Autodesk Inventor part; units mm, degrees
ref_plane "Work Plane1" through (254, 0, 0) normal (1, 0, 0) x (0, 0, -1)
ref_plane "Work Plane2" through (254, 0, 0) normal (1, 0, 0) x (0, 0, -1)
ref_plane "Work Plane3" through (254, 0, 0) normal (1, 0, 0) x (0, 0, -1)
ref_plane "Work Plane1" through (254, 0, 0) normal (1, 0, 0) x (0, 0, -1)
ref_plane "Work Plane2" through (254, 0, 0) normal (1, 0, 0) x (0, 0, -1)
sketch "Sketch3" plane through (254, 0, 0) normal (1, 0, 0) x (0, 0, -1)
  arc A0 (-0.5014, 9.9874) -> (0.4986, 9.9876) centre (0, 0) ccw
  line L0 (0.4986, 9.9876) -> (-0.5014, 9.9874)
  line L1 (-0.5014, 9.9874) -> (-0.7511, 8.9686)
  line L2 (0.4986, 9.9876) -> (0.7489, 8.9688)
  line L3 (-3.0693, 9.5173) -> (-3.0468, 8.4686)
  line L4 (-2.1034, 9.7763) -> (-3.0693, 9.5173)
  line L5 (-2.1034, 9.7763) -> (-1.5979, 8.857)
  line L6 (-5.428, 8.3986) -> (-5.1348, 7.3915)
  line L7 (-4.562, 8.8988) -> (-5.428, 8.3986)
  line L8 (-4.562, 8.8988) -> (-3.8358, 8.1416)
  line L9 (-7.4167, 6.7076) -> (-6.8729, 5.8106)
  line L10 (-6.7097, 7.4148) -> (-7.4167, 6.7076)
  line L11 (-6.7097, 7.4148) -> (-5.8124, 6.8714)
  line L12 (-8.9001, 4.5595) -> (-8.1426, 3.8338)
  line L13 (-8.4002, 5.4256) -> (-8.9001, 4.5595)
  line L14 (-8.4002, 5.4256) -> (-7.3928, 5.1329)
  line L15 (-9.7769, 2.1006) -> (-8.8574, 1.5957)
  line L16 (-9.5182, 3.0666) -> (-9.7769, 2.1006)
  line L17 (-9.5182, 3.0666) -> (-8.4694, 3.0447)
  line L18 (-9.9874, -0.5014) -> (-8.9686, -0.7511)
  line L19 (-9.9876, 0.4986) -> (-9.9874, -0.5014)
  line L20 (-9.9876, 0.4986) -> (-8.9688, 0.7489)
  line L21 (-9.5173, -3.0693) -> (-8.4686, -3.0468)
  line L22 (-9.7763, -2.1034) -> (-9.5173, -3.0693)
  line L23 (-9.7763, -2.1034) -> (-8.857, -1.5979)
  line L24 (-8.3986, -5.428) -> (-7.3915, -5.1348)
  line L25 (-8.8988, -4.562) -> (-8.3986, -5.428)
  line L26 (-8.8988, -4.562) -> (-8.1416, -3.8358)
  line L27 (-6.7076, -7.4167) -> (-5.8106, -6.8729)
  line L28 (-7.4148, -6.7097) -> (-6.7076, -7.4167)
  line L29 (-7.4148, -6.7097) -> (-6.8714, -5.8124)
  line L30 (-4.5595, -8.9001) -> (-3.8338, -8.1426)
  line L31 (-5.4256, -8.4002) -> (-4.5595, -8.9001)
  line L32 (-5.4256, -8.4002) -> (-5.1329, -7.3928)
  line L33 (-2.1006, -9.7769) -> (-1.5957, -8.8574)
  line L34 (-3.0666, -9.5182) -> (-2.1006, -9.7769)
  line L35 (-3.0666, -9.5182) -> (-3.0447, -8.4694)
  line L36 (0.5014, -9.9874) -> (0.7511, -8.9686)
  line L37 (-0.4986, -9.9876) -> (0.5014, -9.9874)
  line L38 (-0.4986, -9.9876) -> (-0.7489, -8.9688)
  line L39 (3.0693, -9.5173) -> (3.0468, -8.4686)
  line L40 (2.1034, -9.7763) -> (3.0693, -9.5173)
  line L41 (2.1034, -9.7763) -> (1.5979, -8.857)
  line L42 (5.428, -8.3986) -> (5.1348, -7.3915)
  line L43 (4.562, -8.8988) -> (5.428, -8.3986)
  line L44 (4.562, -8.8988) -> (3.8358, -8.1416)
  line L45 (7.4167, -6.7076) -> (6.8729, -5.8106)
  line L46 (6.7097, -7.4148) -> (7.4167, -6.7076)
  line L47 (6.7097, -7.4148) -> (5.8124, -6.8714)
  line L48 (8.9001, -4.5595) -> (8.1426, -3.8338)
  line L49 (8.4002, -5.4256) -> (8.9001, -4.5595)
  line L50 (8.4002, -5.4256) -> (7.3928, -5.1329)
  line L51 (9.7769, -2.1006) -> (8.8574, -1.5957)
  line L52 (9.5182, -3.0666) -> (9.7769, -2.1006)
  line L53 (9.5182, -3.0666) -> (8.4694, -3.0447)
  line L54 (9.9874, 0.5014) -> (8.9686, 0.7511)
  line L55 (9.9876, -0.4986) -> (9.9874, 0.5014)
  line L56 (9.9876, -0.4986) -> (8.9688, -0.7489)
  line L57 (9.5173, 3.0693) -> (8.4686, 3.0468)
  line L58 (9.7763, 2.1034) -> (9.5173, 3.0693)
  line L59 (9.7763, 2.1034) -> (8.857, 1.5979)
  line L60 (8.3986, 5.428) -> (7.3915, 5.1348)
  line L61 (8.8988, 4.562) -> (8.3986, 5.428)
  line L62 (8.8988, 4.562) -> (8.1416, 3.8358)
  line L63 (6.7076, 7.4167) -> (5.8106, 6.8729)
  line L64 (7.4148, 6.7097) -> (6.7076, 7.4167)
  line L65 (7.4148, 6.7097) -> (6.8714, 5.8124)
  line L66 (4.5595, 8.9001) -> (3.8338, 8.1426)
  line L67 (5.4256, 8.4002) -> (4.5595, 8.9001)
  line L68 (5.4256, 8.4002) -> (5.1329, 7.3928)
  line L69 (2.1006, 9.7769) -> (1.5957, 8.8574)
  line L70 (3.0666, 9.5182) -> (2.1006, 9.7769)
  line L71 (3.0666, 9.5182) -> (3.0447, 8.4694)
  arc A1 (-0.7511, 8.9686) -> (-1.5979, 8.857) centre (0, 0) ccw
  arc A2 (-3.0468, 8.4686) -> (-3.8358, 8.1416) centre (0, 0) ccw
  arc A3 (-5.1348, 7.3915) -> (-5.8124, 6.8714) centre (0, 0) ccw
  arc A4 (-6.8729, 5.8106) -> (-7.3928, 5.1329) centre (0, 0) ccw
  arc A5 (-8.1426, 3.8338) -> (-8.4694, 3.0447) centre (0, 0) ccw
  arc A6 (-8.8574, 1.5957) -> (-8.9688, 0.7489) centre (0, 0) ccw
  arc A7 (-8.9686, -0.7511) -> (-8.857, -1.5979) centre (0, 0) ccw
  arc A8 (-8.4686, -3.0468) -> (-8.1416, -3.8358) centre (0, 0) ccw
  arc A9 (-7.3915, -5.1348) -> (-6.8714, -5.8124) centre (0, 0) ccw
  arc A10 (-5.8106, -6.8729) -> (-5.1329, -7.3928) centre (0, 0) ccw
  arc A11 (-3.8338, -8.1426) -> (-3.0447, -8.4694) centre (0, 0) ccw
  arc A12 (-1.5957, -8.8574) -> (-0.7489, -8.9688) centre (0, 0) ccw
  arc A13 (0.7511, -8.9686) -> (1.5979, -8.857) centre (0, 0) ccw
  arc A14 (3.0468, -8.4686) -> (3.8358, -8.1416) centre (0, 0) ccw
  arc A15 (5.1348, -7.3915) -> (5.8124, -6.8714) centre (0, 0) ccw
  arc A16 (6.8729, -5.8106) -> (7.3928, -5.1329) centre (0, 0) ccw
  arc A17 (8.1426, -3.8338) -> (8.4694, -3.0447) centre (0, 0) ccw
  arc A18 (8.8574, -1.5957) -> (8.9688, -0.7489) centre (0, 0) ccw
  arc A19 (8.9686, 0.7511) -> (8.857, 1.5979) centre (0, 0) ccw
  arc A20 (8.4686, 3.0468) -> (8.1416, 3.8358) centre (0, 0) ccw
  arc A21 (7.3915, 5.1348) -> (6.8714, 5.8124) centre (0, 0) ccw
  arc A22 (5.8106, 6.8729) -> (5.1329, 7.3928) centre (0, 0) ccw
  arc A23 (3.8338, 8.1426) -> (3.0447, 8.4694) centre (0, 0) ccw
  arc A24 (1.5957, 8.8574) -> (0.7489, 8.9688) centre (0, 0) ccw
  dimension "d24" = 1.5
  dimension "d25" = 1
  dimension "d28" = 360
extrude "Extrusion3" add sketch "Sketch3" against normal blind 10 contours L0 L2 A24 L69 L70 L71 A23 L66 L67 L68 A22 L63 L64 L65 A21 L60 L61 L62 A20 L57 L58 L59 A19 L54 L55 L56 A18 L51 L52 L53 A17 L48 L49 L50 A16 L45 L46 L47 A15 L42 L43 L44 A14 L39 L40 L41 A13 L36 L37 L38 A12 L33 L34 L35 A11 L30 L31 L32 A10 L27 L28 L29 A9 L24 L25 L26 A8 L21 L22 L23 A7 L18 L19 L20 A6 L15 L16 L17 A5 L12 L13 L14 A4 L9 L10 L11 A3 L6 L7 L8 A2 L3 L4 L5 A1 L1
ref_plane "Work Plane3" through (254, 0, 0) normal (1, 0, 0) x (0, 0, -1)
sketch "Sketch4" plane through (254, 0, 0) normal (1, 0, 0) x (0, 0, -1)
  circle A0 centre (0, 0) radius 2.5
  dimension "d32" = 5
extrude "Extrusion4" cut sketch "Sketch4" against normal blind 10
sketch "Sketch5" plane through (0, 0, 0) normal (1, 0, 0) x (0, 1, 0)
  point P0 (0, 0)
properties part number "parte adicional"
Input: part model. Units: mm. Frame: model coordinates. A direction names the side the tool comes from. Give positions to 0.01 mm unless a question says otherwise; leave off trailing zeros. Loops run counter-clockwise (first coordinate to the right, second up) from the corner with the lowest first, then second, coordinate; pieces in that order, holes last. Notation, with made-up numbers: (48.5, -10) - (78.5, -10) arc R14 cw to (78.5, 0) - close; hole circle Ø2 at (-16.75, 69.5). An arc over 180 degrees is marked (long way). Use CSV: the item, a comma, the result in double quotes. Start each with the question number.
Item 1: Reachability of faces 5 (the flat face through (249.07, 1.854, -9.323)), 6 (the flat face through (249.07, 9.32, -1.85)), 7 (the flat face through (249.07, -7.15, -6.27)) from +Z, -Z, +X, -X, +Y, -Y: full face, straight path, thin tool, end or side. Return the list, or none.
Item 2: Contact query for flat-ended pins moving along their axis: P1, Ø6, axis at x = 251.5, y = 7, coming from the -Z side; P2, Ø1, axis at x = 250, z = -6.5, coming from the -Y side; P3, Ø1.5, axis at x = 250.5, y = 3.5, coming from the +Z side. Output: stop coordinate, or through.
Item 3: Line query: line 1 (Z direction, x = 246.25, y = -9); line 2 (Z direction, x = 245, y = 8.25); line 3 (Y direction, x = 250.25, z = 0). Output: solid intervals per line, ascending.
Item 4: Mould query, pull axis Y, two halves, no side actions, for faces 1 (the flat face through (249.07, -6.27, -7.15)), 2 (the flat face through (249.07, -7.9, 5.28)), 3 (the flat face through (249.07, -9.65, -2.58)), 4 (the flat face through (249.07, 9.49, -0.62)). Classes: pulls with the +Y half, pulls with the -Y half, needs draft (parallel to the pull), parting line crosses it, or undercut.
Item 5: Section A-A on z = 0. Return loops of the section in (x, y), then the cut area to 3 significant figures.
Ans:
1,face 5,"-Z, +X, -X"
1,face 6,"+X, -X, +Y"
1,face 7,"+X, -X, -Y"
2,P1,"stops at z = -8.9"
2,P2,"stops at y = -7.41"
2,P3,"stops at z = 9.6"
3,line 1,"z = -3.06 to -1.68, -0.74 to 0.74, 1.67 to 3.06"
3,line 2,"z = -5.38 to -3.94, -3.6 to 3.6, 3.94 to 5.38"
3,line 3,"y = -9.99 to -2.5, 2.5 to 9.99"
4,face 1,"undercut"
4,face 2,"undercut"
4,face 3,"pulls with the -Y half"
4,face 4,"pulls with the +Y half"
5,outline,"(244, -9.99) - (254, -9.99) - (254, -2.5) - (244, -2.5) - close; (244, 2.5) - (254, 2.5) - (254, 9.99) - (244, 9.99) - close"
5,area,"150 mm2"
